For this review, use the dimensioned drawing (mm, ordinates from the lowest corner) and the shaded views. A direction names the side the tool comes from. Round coordinates to 2 decimals unless told otherwise and drop trailing zeros. Write each loop counter-clockwise with the first axis right and the second up, starting at its lowest first coordinate (ties: lowest second). Pieces come first, ordered by that corner, then holes.
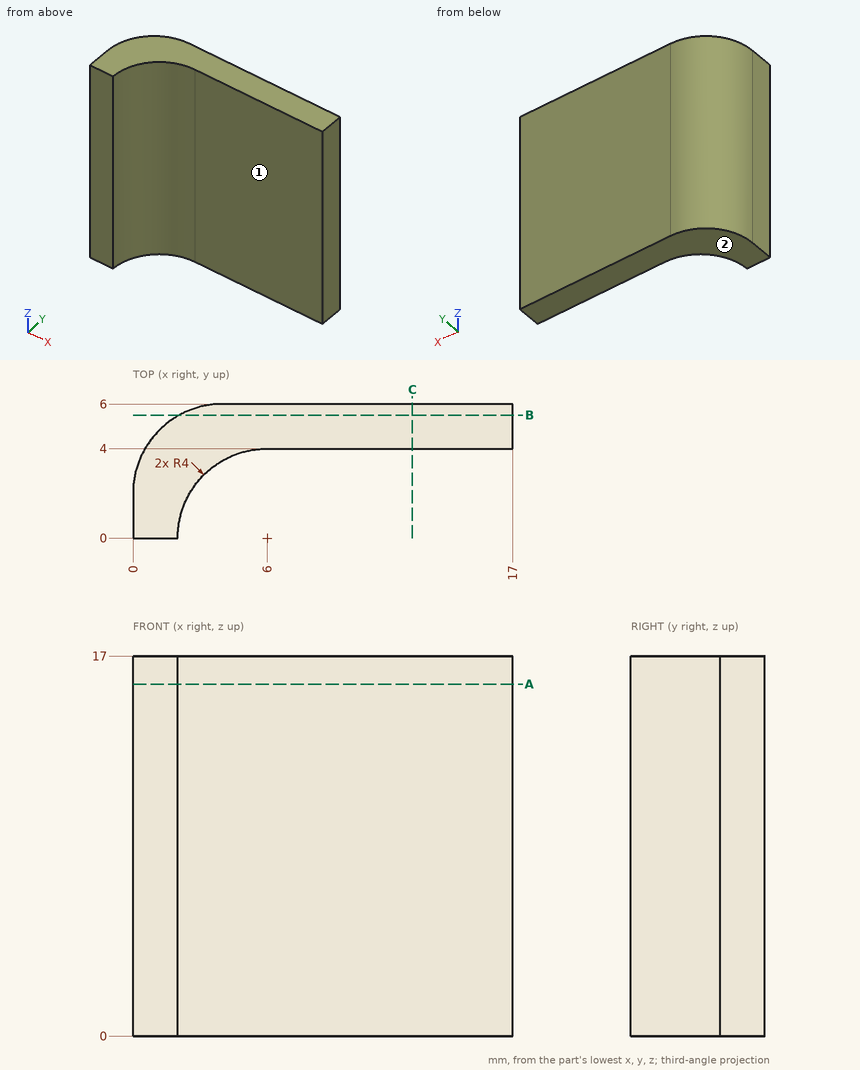
1) For the marked faces 1 and 2, list the 3-axis set-ups (+Z, -Z, +X, -X, +Y, -Y) from which the entire face can be reached by the end or side of a thin tool; tool diameter is ignored.
2) Add section A-A on z = 15.75. State the section outline as (x, y) points, and give its area (3 significant figures).
3) For P1, Ø1.5, axis at y = 4, z = 11.5, coming from the -X side; P2, Ø5, axis at x = 7.5, z = 7, coming from the -Y side; P3, Ø1, axis at y = 5, z = 4.5, coming from the -X side, all flat-tipped, find the tip position at first contact; note any pin that passes through.
4) For line 1 along Y through (x, z) = (16, 11); line 2 along X through (y, z) = (3, 2.5); line 3 along X through (y, z) = (5.5, 2.75), list the stretches that pass through material, from the lowest coordinate up.
5) Add section B-B on y = 5.5. State the section outline as (x, z) points, and give its area (3 significant figures).
6) Add section C-C on x = 12.5. State the section outline as (y, z) points.
Computed:
1. face 1: +Z, -Z, +X, -Y
1. face 2: -Z, +X, -X, +Y, -Y
2. outline: (0, 0) - (2, 0) arc R4 cw to (6, 4) - (17, 4) - (17, 6) - (4, 6) arc R4 ccw to (0, 2) - close
2. area: 42.0 mm2
3. P1: stops at x = 0.2
3. P2: stops at y = 3.87
3. P3: stops at x = 0.88
4. line 1: y = 4 to 6
4. line 2: x = 0.13 to 3.35
4. line 3: x = 2.06 to 17
5. outline: (2.06, 0) - (17, 0) - (17, 17) - (2.06, 17) - close
5. area: 254 mm2
6. outline: (4, 0) - (6, 0) - (6, 17) - (4, 17) - close
